For this review, take the finished solid that the model builds, in its own axes (mm). Face numbers are marked on the shaded views. Round coordinates to 2 decimals unless told otherwise and drop trailing zeros. Order: outer loops, then holes, each group sorted by start corner. A loop starts at its lowest first (then second) coordinate and runs counter-clockwise, first axis right, second up.
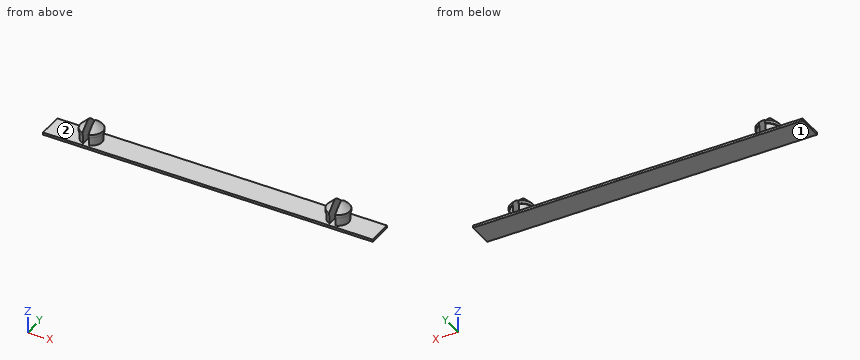
```python
from build123d import *

# Parameters (mm, degrees)
SKICA2_W                 = 55.6
SKICA2_H                 = 4.2
P_IDAT_VYSUNUT_M2_DEPTH  = 0.4
SKICA3_R                 = 1.75
P_IDAT_VYSUNUT_M3_DEPTH  = 1.5
SKICA5_R                 = 1.9
P_IDAT_VYSUNUT_M5_DEPTH  = 2
ZKOSEN_2_SIZE            = 1.5
SKICA7_W                 = 1
SKICA7_H                 = 5
ODEBRAT_VYSUNUT_M1_DEPTH = 3.5


with BuildPart() as part:
    # Skica2 → Přidat vysunutím2 (new body)
    with BuildSketch(Plane.XY):
        Rectangle(SKICA2_W, SKICA2_H)
    extrude(amount=P_IDAT_VYSUNUT_M2_DEPTH)

    # Skica3 → Přidat vysunutím3 (add)
    with BuildSketch(Plane.XY.offset(0.4)):
        with Locations((-20.8, 0)):
            Circle(SKICA3_R)
        with Locations((20.8, 0)):
            Circle(SKICA3_R)
    extrude(amount=P_IDAT_VYSUNUT_M3_DEPTH)

    # Skica5 → Přidat vysunutím5 (add)
    with BuildSketch(Plane.XY.offset(1.9)):
        with Locations((-20.8, 0)):
            Circle(SKICA5_R)
        with Locations((20.8, 0)):
            Circle(SKICA5_R)
    extrude(amount=P_IDAT_VYSUNUT_M5_DEPTH)

    # Zkosení2
    zkosen_2_edges = [part.edges().sort_by_distance(p)[0] for p in [
        (-22.7, 0, 3.9),
        (18.9, 0, 3.9),
    ]]
    chamfer(zkosen_2_edges, length=ZKOSEN_2_SIZE)

    # Skica7 → Odebrat vysunutím1 (cut)
    with BuildSketch(Plane.XY.offset(3.9)):
        with Locations((-20.8, 0)):
            Rectangle(SKICA7_W, SKICA7_H)
        with Locations((20.8, 0)):
            Rectangle(SKICA7_W, SKICA7_H)
    extrude(amount=-ODEBRAT_VYSUNUT_M1_DEPTH, mode=Mode.SUBTRACT)


solid = part.part
```
Q1. Take a section at B-B, the plane x = 6. State the section outline as (y, z) points.
Q2. Clearance check with flat-ended pins moving along their axes: pin 1 (0.7 mm diameter, centred on x = -22, y = 1, fed in from -Z); pin 2 (1.7 mm diameter, centred on y = 0.5, z = 2.5, fed in from -X); pin 3 (1.5 mm diameter, centred on x = -21.5, z = 2.5, fed in from -Y); pin 4 (2 mm diameter, centred on x = -7, z = 2, fed in from +Y). State where each tip first meets the part, or that it passes through.
Q3. Take a section at A-A, the plane z = 1.1. State the section outline as (x, y) points.
Q4. Mouldability with a two-part tool opening along X and no side actions: class the marked faces 1 and 2 as +X half, -X half, draft (parallel to the pull), parting line (faces both ways), or undercut.
Q5. Wall thickness on line 1 (X direction, y = 1.3, z = 1.7); line 2 (X direction, y = 0.5, z = 3.3); line 3 (Z direction, x = -6, y = -0.35): over which ranges is each line inside the solid? List them lowest first.
Working result:
1. outline: (-2.1, 0) - (2.1, 0) - (2.1, 0.4) - (-2.1, 0.4) - close
2. pin 1: stops at z = 0
2. pin 2: stops at x = -22.7
2. pin 3: stops at y = -1.83
2. pin 4: passes through
3. outline: (-21.3, -1.68) - (-21.3, 1.68) arc R1.75 ccw to start; (-20.3, -1.68) arc R1.75 ccw to (-20.3, 1.68) - close; (20.3, -1.68) - (20.3, 1.68) arc R1.75 ccw to start; (21.3, -1.68) arc R1.75 ccw to (21.3, 1.68) - close
4. face 1: draft
4. face 2: undercut
5. line 1: x = -21.97 to -21.3, -20.3 to -19.63, 19.63 to 20.3, 21.3 to 21.97
5. line 2: x = -21.67 to -21.3, -20.3 to -19.93, 19.93 to 20.3, 21.3 to 21.67
5. line 3: z = 0 to 0.4
